```python
from build123d import *

# Parameters (mm, degrees)
SKETCH_1_W          = 50
SKETCH_1_H          = 48
EXTRUDE_1_DEPTH     = 25
SKETCH_2_R          = 10.5
CUT_EXTRUDE_1_DEPTH = 26
CHAMFER_1_SIZE      = 6
CHAMFER_1_SIZE2     = 10.392304845
CHAMFER_2_SIZE      = 6
CHAMFER_2_SIZE2     = 10.392304845


with BuildPart() as part:
    # Эскиз1 → Бобышка-Вытянуть1 (new body)
    with BuildSketch(Plane.XY):
        with Locations((25, 24)):
            Rectangle(SKETCH_1_W, SKETCH_1_H)
    extrude(amount=EXTRUDE_1_DEPTH)

    # Эскиз2 → Вырез-Вытянуть1 (cut, through all)
    with BuildSketch(Plane.XY.offset(25)):
        with Locations((25, 23)):
            Circle(SKETCH_2_R)
    extrude(amount=-CUT_EXTRUDE_1_DEPTH, mode=Mode.SUBTRACT)

    # Фаска1
    chamfer_1_edges = [part.edges().sort_by_distance(p)[0] for p in [
        (25, 0, 0),
    ]]
    chamfer_1_side = [part.faces().sort_by_distance(p)[0] for p in [
        (25, 0.693108938, 0),
    ]]
    chamfer(chamfer_1_edges, length=CHAMFER_1_SIZE, length2=CHAMFER_1_SIZE2, reference=chamfer_1_side[0])

    # Фаска2
    chamfer_2_edges = [part.edges().sort_by_distance(p)[0] for p in [
        (25, 0, 25),
    ]]
    chamfer_2_side = [part.faces().sort_by_distance(p)[0] for p in [
        (25, 0.693108938, 25),
    ]]
    chamfer(chamfer_2_edges, length=CHAMFER_2_SIZE, length2=CHAMFER_2_SIZE2, reference=chamfer_2_side[0])


solid = part.part
```
Input: part model. Units: mm. Frame: model coordinates. Give positions to 0.01 mm unless a question says otherwise; leave off trailing zeros. Order: outer loops, then holes, each group sorted by start corner. A loop starts at its lowest first (then second) coordinate and runs counter-clockwise, first axis right, second up. Notation, with made-up numbers: M -38,60 L -34,60 A25 ccw -34,73 Z; hole C 64.5,86 d3. An arc over 180 degrees is marked long. One line per question, with ' | ' between items.
1) Contact query for a flat-ended pin moving along its axis: P1, Ø8, axis at x = 37.5, z = 20, coming from the -Y side. Output: stop coordinate, or through.
Filled in:
P1: stops at y = 0.8
2) Section B-B on z = 13. Output: boundary loops of the cut face in (x, y).
Filled in:
outline: M 0,0 L 50,0 L 50,48 L 0,48 Z; hole C 25,23 d21
3) Draft query along X for faces 1 (the face through (0, 24, 12)), 2 (the face through (17.261, 30.096, 12.675)), 3 (the face through (19, 32, 0)). Return one class per face: pulls with the +X half, pulls with the -X half, needs draft (parallel to the pull), parting line crosses it, or undercut.
Filled in:
face 1: pulls with the -X half | face 2: undercut | face 3: needs draft
4) Ray query, L1, parallel to Y at x = 25, z = 10.75; L2, parallel to Y at x = 22, z = 24.25; L3, parallel to X at y = 30.5, z = 2.5. Return the intervals inside material, ascending.
Filled in:
L1: y = 0 to 12.5, 33.5 to 48 | L2: y = 5.57 to 12.94, 33.06 to 48 | L3: x = 0 to 17.65, 32.35 to 50
5) Section C-C on y = 23. Output: boundary loops of the cut face in (x, z), and give its area (3 significant figures).
Filled in:
outline: M 0,0 L 14.5,0 L 14.5,25 L 0,25 Z; M 35.5,0 L 50,0 L 50,25 L 35.5,25 Z | area: 725 mm2
6) Section D-D on x = 7.5. Output: boundary loops of the cut face in (y, z), and give its area (3 significant figures).
Filled in:
outline: M 0,10.39 L 6,0 L 48,0 L 48,25 L 6,25 L 0,14.61 Z | area: 1,140 mm2
7) Section A-A on x = 25. Output: boundary loops of the cut face in (y, z).
Filled in:
outline: M 0,10.39 L 6,0 L 12.5,0 L 12.5,25 L 6,25 L 0,14.61 Z; M 33.5,0 L 48,0 L 48,25 L 33.5,25 Z
